Autodesk Inventor part; units mm, degrees
ref_plane "YZ Plane" through (0, 0, 0) normal (1, 0, 0) x (0, 1, 0)
ref_plane "XZ Plane" through (0, 0, 0) normal (0, 1, 0) x (-1, 0, 0)
ref_plane "XY Plane" through (0, 0, 0) normal (0, 0, 1) x (1, 0, 0)
sketch "스케치1" plane through (0, 0, 0) normal (0, 1, 0) x (-1, 0, 0)
  line L0 (0, 0) -> (-8.1, 0)
  line L1 (-8.1, 0) -> (-21.65, 15.7)
  line L2 (-21.65, 15.7) -> (-21.65, 8.0474)
  line L3 (-21.65, 8.0474) -> (-10.3894, -5)
  line L4 (-10.3894, -5) -> (0, -5)
  line L5 (0, -5) -> (0, 0)
  line L6 (0, 0) -> (8.1, 0)
  line L7 (8.1, 0) -> (21.65, 15.7)
  line L8 (21.65, 15.7) -> (21.65, 8.0474)
  line L9 (21.65, 8.0474) -> (10.3894, -5)
  line L10 (10.3894, -5) -> (0, -5)
  dimension "d0" = 15.7
  dimension "d1" = 43.3
  dimension "d2" = 16.2
  dimension "d3" = 5
  dimension "d4" = 5
extrude "돌출1" add sketch "스케치1" along normal blind 20
sketch "스케치2" plane through (21.65, 0, 15.7) normal (-0.757, 0, 0.6534) x (0.6534, 0, 0.757)
  line L0 (-20.7387, 20) -> (0, 20)
  line L1 (-9.7387, 20) -> (-9.7387, 0)
  line L2 (-20.7387, 0) -> (0, 0)
  line L3 (0, 0) -> (0, 20)
  line L4 (-20.7387, 0) -> (-20.7387, 20)
  circle A0 centre (-9.7387, 10) radius 1.75
  point P0 (-26.031, 0)
  dimension "d8" = 11
  dimension "d9" = 3.5
  dimension "d10" = 10
  dimension "d11" = 11
extrude "돌출2" cut sketch "스케치2" against normal through all contours A0 L1 | L1 A0
mirror "미러1" about plane through (0, 0, 0) normal (1, 0, 0) of "돌출2"
chamfer "모따기1" distance 5 angle 45 4 edges at (16.0197, 20, 1.5237) (-16.0197, 20, 1.5237) (16.0197, 0, 1.5237) (-16.0197, 0, 1.5237)
properties part number "sun3" material "티타늄"
For this review, take the finished solid that the model builds, in its own axes (mm). A direction names the side the tool comes from. Give positions to 0.01 mm unless a question says otherwise; leave off trailing zeros. Loops run counter-clockwise (first coordinate to the right, second up) from the corner with the lowest first, then second, coordinate; pieces in that order, holes last. Notation, with made-up numbers: M 48,67 L 92,67 A19 ccw 92,85 Z; hole C -14,4 d11. An arc over 180 degrees is marked long. Put each result on its own line as item: value. Start each with the question number.
(1) Add section A-A, the plane z = 12. Write out the cut boundary in (x, y).
(2) Wall thickness on L1, parallel to Z at x = -1.5, y = 12.5; L2, parallel to X at y = 15, z = 0.5; L3, parallel to X at y = 7, z = 11.25: over which ranges is each line inside the solid? List them lowest first.
(3) Add section C-C, the plane y = 13. Write out the cut boundary in (x, z), then the cut area to 3 significant figures.
(4) Add section B-B, the plane y = 8.75. Write out the cut boundary in (x, z), then the cut area to 3 significant figures.
(5) The part is to be moulded in two halves that separate along X. For faces 1 (the flat face through (0, 20, -2)), 2 (the cylindrical face through (-17.004, 8.265, 6.544)), 3 (the flat face through (21.65, 10, 13)), say which applies: +X half, -X half, draft (parallel to the pull), parting line (faces both ways), or undercut.
(6) Machinability: for faces 4 (the flat face through (-14.458, 2.465, 3.595)), 5 (the flat face through (-14.78, 12.08, 7.74)), which of the approach directions +Z, -Z, +X, -X, +Y, -Y give a long, thin tool a straight path to every point of the face, cutting with its end or side? Answer none if there is none.
(7) For pin 1 (4 mm diameter, centred on x = 14, y = 16, fed in from +Z); pin 2 (6 mm diameter, centred on x = 10, y = 4, fed in from +Z); pin 3 (4 mm diameter, centred on x = -16, y = 7, fed in from -Z), all flat-tipped, find the tip position at first contact; note any pin that passes through.
(8) Add section D-D, the plane x = -7. Write out the cut boundary in (y, z), then the cut area to 3 significant figures.
Result:
1. outline: M -21.65,2.42 L -18.46,0 L -18.46,20 L -21.65,17.58 Z; M 18.46,0 L 21.65,2.42 L 21.65,17.58 L 18.46,20 Z
2. L1: z = -5 to 0
2. L2: x = -15.14 to -8.53, 8.53 to 15.14
2. L3: x = -21.65 to -17.81, 17.81 to 21.65
3. outline: M -21.65,8.05 L -10.39,-5 L 10.39,-5 L 21.65,8.05 L 21.65,15.7 L 8.1,0 L -8.1,0 L -21.65,15.7 Z
3. area: 282 mm^2
4. outline: M -21.65,8.05 L -19.87,5.99 L -16.09,9.25 L -21.65,15.7 Z; M -18.27,4.13 L -10.39,-5 L 10.39,-5 L 18.27,4.13 L 14.49,7.4 L 8.1,0 L -8.1,0 L -14.49,7.4 Z; M 16.09,9.25 L 19.87,5.99 L 21.65,8.05 L 21.65,15.7 Z
4. area: 258 mm^2
5. face 1: draft
5. face 2: undercut
5. face 3: +X half
6. face 4: -Z, -X, -Y
6. face 5: +Z, +Y, -Y
7. pin 1: stops at z = 9.15
7. pin 2: stops at z = 5.68
7. pin 3: stops at z = -0.82
8. outline: M 0,-1.27 L 2.43,-5 L 17.57,-5 L 20,-1.27 L 20,0 L 0,0 Z
8. area: 90.9 mm^2
